from build123d import *

# Parameters (mm, degrees)
SKETCH_1_W      = 26
SKETCH_1_H      = 26
SKETCH_1_R      = 1.1
EXTRUDE_1_DEPTH = 3
SKETCH_2_W      = 32
SKETCH_2_H      = 26
SKETCH_2_R      = 1.1
EXTRUDE_2_DEPTH = 2
EXTRUDE_START   = 2
SKETCH_3_W      = 32
SKETCH_3_H      = 26
SKETCH_3_R      = 1.1
EXTRUDE_3_DEPTH = 2


with BuildPart() as part:
    # ｽｹｯﾁ1 → ﾎﾞｽ - 押し出し1 (new body)
    with BuildSketch(Plane.XY):
        Rectangle(SKETCH_1_W, SKETCH_1_H)
        with Locations((1.45, 0)):
            Circle(SKETCH_1_R, mode=Mode.SUBTRACT)
        with Locations((1.45, 6)):
            Circle(SKETCH_1_R, mode=Mode.SUBTRACT)
        with Locations((5.692640687, 4.242640687)):
            Circle(SKETCH_1_R, mode=Mode.SUBTRACT)
        with Locations((7.45, 0)):
            Circle(SKETCH_1_R, mode=Mode.SUBTRACT)
        with Locations((5.692640687, -4.242640687)):
            Circle(SKETCH_1_R, mode=Mode.SUBTRACT)
        with Locations((1.45, -6)):
            Circle(SKETCH_1_R, mode=Mode.SUBTRACT)
        with Locations((-2.792640687, -4.242640687)):
            Circle(SKETCH_1_R, mode=Mode.SUBTRACT)
        with Locations((-4.55, 0)):
            Circle(SKETCH_1_R, mode=Mode.SUBTRACT)
        with Locations((-2.792640687, 4.242640687)):
            Circle(SKETCH_1_R, mode=Mode.SUBTRACT)
    extrude(amount=EXTRUDE_1_DEPTH)

    # ｽｹｯﾁ2 → ﾎﾞｽ - 押し出し2 (add)
    with BuildSketch(Plane.ZY.offset(13)):
        with Locations((16, 0)):
            Rectangle(SKETCH_2_W, SKETCH_2_H)
        with Locations((29.5, 10.5)):
            Circle(SKETCH_2_R, mode=Mode.SUBTRACT)
        with Locations((8.5, 10.5)):
            Circle(SKETCH_2_R, mode=Mode.SUBTRACT)
        with Locations((8.5, -10.5)):
            Circle(SKETCH_2_R, mode=Mode.SUBTRACT)
        with Locations((29.5, -10.5)):
            Circle(SKETCH_2_R, mode=Mode.SUBTRACT)
    extrude(amount=EXTRUDE_2_DEPTH)

    # ｽｹｯﾁ3 → ﾎﾞｽ - 押し出し3 (add)
    with BuildSketch(Plane(origin=(13, 0, 0), x_dir=(0, 0, -1), z_dir=(1, 0, 0)).offset(EXTRUDE_START)):
        with Locations((-16, 0)):
            Rectangle(SKETCH_3_W, SKETCH_3_H)
        with Locations(Location((-8.5, -10.5, 0), (0, 0, 180))):
            Circle(SKETCH_3_R, mode=Mode.SUBTRACT)
        with Locations(Location((-8.5, 10.5, 0), (0, 0, 180))):
            Circle(SKETCH_3_R, mode=Mode.SUBTRACT)
        with Locations(Location((-29.5, 10.5, 0), (0, 0, 180))):
            Circle(SKETCH_3_R, mode=Mode.SUBTRACT)
        with Locations(Location((-29.5, -10.5, 0), (0, 0, 180))):
            Circle(SKETCH_3_R, mode=Mode.SUBTRACT)
    extrude(amount=-EXTRUDE_3_DEPTH)


solid = part.part
Here's how the part is built. I have some questions about the finished solid (model axes, mm). Round coordinates to 2 decimals unless told otherwise and drop trailing zeros. Loops run counter-clockwise (first coordinate to the right, second up) from the corner with the lowest first, then second, coordinate; pieces in that order, holes last. Notation, with made-up numbers: (-35.75, -34) -> (2.25, -34) arc R28 ccw to (2.25, -6) -> close; hole circle Ø11 at (-26, -24). An arc over 180 degrees is marked (long way). Write each question's results on one line, items separated by ' | '.
(1) If we section it at C-C, the plane z = 29.5: List the corners of the cut face in (x, y) for me, then the cut area to 3 significant figures.
Worked answers:
outline: (-15, -13) -> (-13, -13) -> (-13, -11.6) -> (-15, -11.6) -> close; (-15, -9.4) -> (-13, -9.4) -> (-13, 9.4) -> (-15, 9.4) -> close; (-15, 11.6) -> (-13, 11.6) -> (-13, 13) -> (-15, 13) -> close; (13, -13) -> (15, -13) -> (15, -11.6) -> (13, -11.6) -> close; (13, -9.4) -> (15, -9.4) -> (15, 9.4) -> (13, 9.4) -> close; (13, 11.6) -> (15, 11.6) -> (15, 13) -> (13, 13) -> close | area: 86.4 mm2
(2) If I drill on L1, parallel to Y at x = 13.7, z = 8.5; L2, parallel to Y at x = 7.45, z = 1.75; L3, parallel to Y at x = 1.45, z = 1.6, over which ranges is the centre line in solid material (lowest first)?
Worked answers:
L1: -13 to -11.6, -9.4 to 9.4, 11.6 to 13 | L2: -13 to -1.1, 1.1 to 13 | L3: -13 to -7.1, -4.9 to -1.1, 1.1 to 4.9, 7.1 to 13
(3) If we section it at D-D, the plane y = 0: List the corners of the cut face in (x, z) for me.
Worked answers:
outline: (-15, 0) -> (-5.65, 0) -> (-5.65, 3) -> (-13, 3) -> (-13, 32) -> (-15, 32) -> close; (-3.45, 0) -> (0.35, 0) -> (0.35, 3) -> (-3.45, 3) -> close; (2.55, 0) -> (6.35, 0) -> (6.35, 3) -> (2.55, 3) -> close; (8.55, 0) -> (15, 0) -> (15, 32) -> (13, 32) -> (13, 3) -> (8.55, 3) -> close
(4) If we section it at A-A, the plane z = 25.5: List the corners of the cut face in (x, y) for me, then the cut area to 3 significant figures.
Worked answers:
outline: (-15, -13) -> (-13, -13) -> (-13, 13) -> (-15, 13) -> close; (13, -13) -> (15, -13) -> (15, 13) -> (13, 13) -> close | area: 104 mm2
(5) We'd pull the mould along Y, two halves only. Please class faces 1 (the face through (15, 0, 16)), 2 (the face through (2.5, -5.67, 1.48)), 3 (the face through (-2, 13, 2)), 4 (the face through (5.549, 5.333, 1.479)): released by +Y, released by -Y, zero draft, split by the parting line, or undercut.
Worked answers:
face 1: zero draft | face 2: undercut | face 3: released by +Y | face 4: undercut
(6) For P1, Ø3, axis at x = -2.79, y = -4.24, coming from the +Z side, with a flat end and sliding along its axis, tell me the tip position at first contact or that it passes through.
Worked answers:
P1: z = 3
(7) If we section it at B-B, the plane x = 1.45: List the corners of the cut face in (y, z) for me, then the cut area to 3 significant figures.
Worked answers:
outline: (-13, 0) -> (-7.1, 0) -> (-7.1, 3) -> (-13, 3) -> close; (-4.9, 0) -> (-1.1, 0) -> (-1.1, 3) -> (-4.9, 3) -> close; (1.1, 0) -> (4.9, 0) -> (4.9, 3) -> (1.1, 3) -> close; (7.1, 0) -> (13, 0) -> (13, 3) -> (7.1, 3) -> close | area: 58.2 mm2
